from build123d import *

# Parameters (mm, degrees)
F1_DEPTH = 4
F2_R     = 0.5
F3_DEPTH = 25
F2_R_2   = 1.05
F4_DEPTH = 10
F2_W     = 20
F2_H     = 8
F5_DEPTH = 6
F6_W     = 8
F6_H     = 2
F7_DEPTH = 6.1
F9_DEPTH = 8


with BuildPart() as f1:
    # F0 (on Front) → F1 (new body, symmetric)
    with BuildSketch(Plane.XZ):
        Polygon((-10, 5), (-10, -5), (-3.135451, -5), (3.135451, -5), (10, -5), (10, 5), align=None)
        with BuildLine():
            Line((10, -5), (3.135451, -5))
            ThreePointArc((3.135451, -5), (4.159274, -5.550715), (4.549477, -6.645814))
            ThreePointArc((4.549477, -6.645814), (1.298147, -10.123692), (0.029146, -14.712418))
            Line((0.029146, -14.712418), (1.529146, -14.712418))
            ThreePointArc((1.529146, -14.712418), (4.260677, -9.20442), (10, -7))
            Line((10, -7), (10, -5))
        make_face()
        with BuildLine():
            Line((-3.135451, -5), (-10, -5))
            Line((-10, -5), (-10, -7))
            ThreePointArc((-10, -7), (-4.260677, -9.20442), (-1.529146, -14.712418))
            Line((-1.529146, -14.712418), (-0.029146, -14.712418))
            ThreePointArc((-0.029146, -14.712418), (-1.298147, -10.123692), (-4.549477, -6.645814))
            ThreePointArc((-4.549477, -6.645814), (-4.159274, -5.550715), (-3.135451, -5))
        make_face()
    extrude(amount=F1_DEPTH, both=True)

    # F2 (on face) → F3 (cut)
    with BuildSketch(Plane.XY.offset(5)):
        Circle(F2_R)
    extrude(amount=-F3_DEPTH, mode=Mode.SUBTRACT)

    # F2 (on face) → F4 (cut)
    with BuildSketch(Plane.XY.offset(5)):
        Circle(F2_R_2)
        Circle(F2_R, mode=Mode.SUBTRACT)
    extrude(amount=-F4_DEPTH, mode=Mode.SUBTRACT)

    # F2 (on face) → F5 (cut)
    with BuildSketch(Plane.XY.offset(5)):
        Rectangle(F2_W, F2_H)
        Circle(F2_R_2, mode=Mode.SUBTRACT)
    extrude(amount=-F5_DEPTH, mode=Mode.SUBTRACT)

    # F6 (on face) → F7 (join)
    with BuildSketch(Plane.YZ.offset(10)):
        with Locations((0, -2)):
            Rectangle(F6_W, F6_H)
    extrude(amount=F7_DEPTH)

    # F8 (on face) → F9 (join)
    with BuildSketch(Plane(origin=(0, 4, 0), x_dir=(-1, 0, 0), z_dir=(0, 1, 0))):
        Polygon((-15.105671, -11.829939), (-16.1, -3), (-16.1, -1), (-18.428246, -1), (-17.105671, -11.829939), align=None)
    extrude(amount=-F9_DEPTH)


solid = f1.part
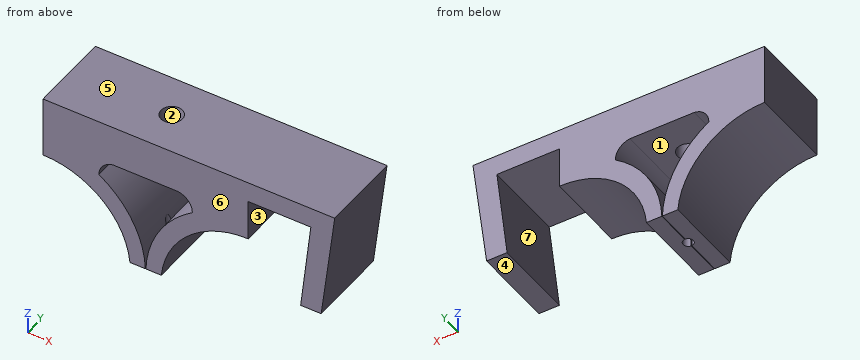
Input: part model. Units: mm. Frame: model coordinates. Face numbers are marked on the shaded views. A direction names the side the tool comes from. Round coordinates to 2 decimals unless told otherwise and drop trailing zeros. Loops run counter-clockwise (first coordinate to the right, second up) from the corner with the lowest first, then second, coordinate; pieces in that order, holes last. Notation, with made-up numbers: (67.5, 64.5) -> (112.5, 64.5) arc R32 cw to (112.5, 97.5) -> close; hole circle Ø5 at (67.25, 6). An arc over 180 degrees is marked (long way). Answer as a JSON object with one key per item and string values. Group by question number.
1) Pin query (flat end, axial travel): pin 1 (3 mm diameter, centred on x = 13.5, y = 0.5, fed in from -Z); pin 2 (2 mm diameter, centred on y = -2, z = -4.5, fed in from +X); pin 3 (1 mm diameter, centred on x = 16, y = -0.5, fed in from -Z). Return the tip coordinate at first contact, or that it passes through.
2) Section query B-B on z = -12.25. Output: boundary loops of the cut face in (x, y).
3) Reachability of the marked faces 1, 2, 3 and 4 from +Z, -Z, +X, -X, +Y, -Y: full face, straight path, thin tool, end or side. Return the list, or none.
4) Section query D-D on z = -8.25. Output: boundary loops of the cut face in (x, y).
5) Ray query, L1, parallel to Y at x = 0, z = -3.4; L2, parallel to X at y = -3, z = -6.75; L3, parallel to X at y = 2.75, z = -6. Return the intervals inside material, ascending.
6) Section query A-A on y = 0. Output: boundary loops of the cut face in (x, z) (3 decimals).
7) Section query C-C on x = -3.5. Output: boundary loops of the cut face in (y, z).
8) Draft query along Z for the marked faces 5, 6 and 7. Return one class per face: +Z half, -Z half, draft (parallel to the pull), parting line (faces both ways), or undercut.
Reply:
{
 "1": {"pin 1": "stops at z = -3", "pin 2": "stops at x = 18.12", "pin 3": "stops at z = -11.83"},
 "2": {"outline": "(-2.13, -4) -> (-0.41, -4) -> (-0.41, -0.28) arc R0.5 cw to (-0.41, 0.28) -> (-0.41, 4) -> (-2.13, 4) -> close; (0.41, -4) -> (2.13, -4) -> (2.13, 4) -> (0.41, 4) -> (0.41, 0.28) arc R0.5 cw to (0.41, -0.28) -> close"},
 "3": {"face 1": "+Y, -Y", "face 2": "+Z", "face 3": "-Z, +Y, -Y", "face 4": "-Z, +X, +Y, -Y"},
 "4": {"outline": "(-5.53, -4) -> (-2.66, -4) -> (-2.66, 4) -> (-5.53, 4) -> close; (2.66, -4) -> (5.53, -4) -> (5.53, 4) -> (2.66, 4) -> close; (15.51, -4) -> (17.54, -4) -> (17.54, 4) -> (15.51, 4) -> close"},
 "5": {"L1": "y = -4 to -1.05, 1.05 to 4", "L2": "x = -10 to -4.39, 4.39 to 10, 15.68 to 17.73", "L3": "x = -10 to -4.43, 4.43 to 10, 15.76 to 17.82"},
 "6": {"outline": "(-10, -7) arc R8.461 cw to (-1.529, -14.712) -> (-0.5, -14.712) -> (-0.5, -11.959) arc R9.975 ccw to (-4.549, -6.646) arc R1.618 cw to (-3.135, -5) -> (-1.05, -5) -> (-1.05, -1) -> (-10, -1) -> close; (0.5, -14.712) -> (1.529, -14.712) arc R8.461 cw to (10, -7) -> (10, -3) -> (16.1, -3) -> (15.106, -11.83) -> (17.106, -11.83) -> (18.428, -1) -> (1.05, -1) -> (1.05, -5) -> (3.135, -5) arc R1.618 cw to (4.549, -6.646) arc R9.975 ccw to (0.5, -11.959) -> close"},
 "7": {"outline": "(-4, -9.99) -> (4, -9.99) -> (4, -7.43) -> (-4, -7.43) -> close; (-4, -5.09) -> (4, -5.09) -> (4, -1) -> (-4, -1) -> close"},
 "8": {"face 5": "+Z half", "face 6": "draft", "face 7": "undercut"}
}
